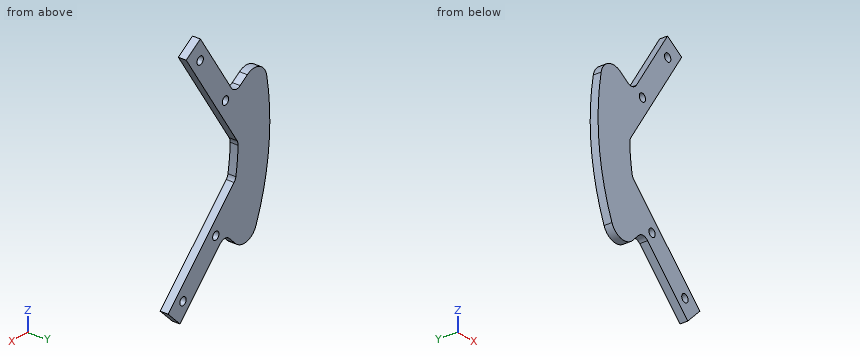
```python
from build123d import *

# Parameters (mm, degrees)
SKETCH1_R           = 1.5
BOSS_EXTRUDE1_DEPTH = 3
FILLET1_R           = 6
FILLET2_R           = 3


with BuildPart() as part:
    # Sketch1 → Boss-Extrude1 (new body)
    with BuildSketch(Plane(origin=(0, 0, 0), x_dir=(1, 0, 0), z_dir=(0, 1, 0))):
        with BuildLine():
            Line((-74.629040009, 40.687914512), (-63.639610307, 29.69848481))
            Line((-63.639610307, 29.69848481), (-42.426406871, 50.911688245))
            Line((-42.426406871, 50.911688245), (-36.769552622, 45.254833996))
            Line((-36.769552622, 45.254833996), (-68.72500623, 13.299380388))
            ThreePointArc((-68.72500623, 13.299380388), (-69.616532676, 7.316992429), (-69.988296617, 1.279975229))
            Line((-69.988296617, 1.279975229), (-45.375058731, -36.621087439))
            Line((-45.375058731, -36.621087439), (-52.084423274, -40.978199719))
            Line((-52.084423274, -40.978199719), (-68.423594325, -15.81808268))
            Line((-68.423594325, -15.81808268), (-81.457709532, -24.282536066))
            ThreePointArc((-81.457709532, -24.282536066), (-84.534361106, 8.884919378), (-74.629040009, 40.687914512))
        make_face()
        with Locations((-43.840620434, 43.840620434)):
            Circle(SKETCH1_R, mode=Mode.SUBTRACT)
        with Locations((-59.39696962, 28.284271247)):
            Circle(SKETCH1_R, mode=Mode.SUBTRACT)
        with Locations((-51.997575213, -33.767620171)):
            Circle(SKETCH1_R, mode=Mode.SUBTRACT)
        with Locations((-63.979633983, -15.316867676)):
            Circle(SKETCH1_R, mode=Mode.SUBTRACT)
    extrude(amount=BOSS_EXTRUDE1_DEPTH)

    # Fillet1
    fillet1_edges = [part.edges().sort_by_distance(p)[0] for p in [
        (-74.629040009, 1.5, -40.687914512),
        (-81.457709532, 1.5, 24.282536066),
    ]]
    fillet(fillet1_edges, radius=FILLET1_R)

    # Fillet2
    fillet2_edges = [part.edges().sort_by_distance(p)[0] for p in [
        (-63.639610307, 1.5, -29.69848481),
        (-68.72500623, 1.5, -13.299380388),
        (-69.988296617, 1.5, -1.279975229),
        (-68.423594325, 1.5, 15.81808268),
    ]]
    fillet(fillet2_edges, radius=FILLET2_R)


solid = part.part
```
Geometry check sheet. Reference: the model listing, model coordinates, mm. Round coordinates to 2 decimals unless told otherwise and drop trailing zeros. Loops run counter-clockwise (first coordinate to the right, second up) from the corner with the lowest first, then second, coordinate; pieces in that order, holes last. Notation, with made-up numbers: (-1, 49) - (46, 49) arc R10 ccw to (46, 67) - close; hole circle Ø2 at (-31.75, 25.5). An arc over 180 degrees is marked (long way). Write each question's results on one line, items separated by ' | '. Start each with the question number.
Q1. Cross-section at B-B on y = 0.6. Enter the section's corners in (x, z), and give its area (3 significant figures).
Q2. Thickness scan on line 1 (Z direction, x = -46, y = 0.55); line 2 (X direction, y = 1.95, z = 15); line 3 (X direction, y = 1.15, z = -29). Record the ranges inside material, lowest first. Write a range as [from, to].
Q3. Cross-section at D-D on z = 24. Enter the section's corners in (x, y).
Q4. Gauge pin test, flat end, axial feed: P1, Ø1.5, axis at x = -47.5, y = 1.5, coming from the +Z side. Record the tip position at first contact, or that the pin passes through.
Q5. Cross-section at C-C on z = -10.5. Enter the section's corners in (x, y).
Q6. Cross-section at A-A on x = -54.5. Enter the section's corners in (y, z).
Answers below:
1) outline: (-83.53, 15.76) arc R85 ccw to (-78.43, -32.78) arc R6 ccw to (-68.65, -34.71) - (-65.76, -31.82) arc R3 cw to (-61.52, -31.82) - (-42.43, -50.91) - (-36.77, -45.25) - (-68.07, -13.96) arc R3 cw to (-68.9, -12.37) arc R70 cw to (-69.96, -2.23) arc R3 cw to (-69.48, -0.5) - (-45.38, 36.62) - (-52.08, 40.98) - (-66.79, 18.33) arc R3 cw to (-70.94, 17.45) - (-74.36, 19.68) arc R6 ccw to start; hole circle Ø3 at (-63.98, 15.32); hole circle Ø3 at (-59.4, -28.28); hole circle Ø3 at (-52, 33.77); hole circle Ø3 at (-43.84, -43.84) | area: 1,400 mm²
2) line 1: z = [-47.34, -36.02], [35.66, 37.03] | line 2: x = [-83.67, -65.45], [-62.51, -59.42] | line 3: x = [-79.9, -60.72], [-58.08, -53.02]
3) outline: (-63.11, 0) - (-53.57, 0) - (-53.57, 3) - (-63.11, 3) - close
4) P1: stops at z = 38.49
5) outline: (-84.35, 0) - (-69.21, 0) - (-69.21, 3) - (-84.35, 3) - close
6) outline: (0, -38.84) - (3, -38.84) - (3, -27.52) - (0, -27.52) - close; (0, 22.57) - (3, 22.57) - (3, 37.26) - (0, 37.26) - close
